Autodesk Inventor part; units mm, degrees
ref_plane "YZ Plane" through (0, 0, 0) normal (1, 0, 0) x (0, 1, 0)
ref_plane "XZ Plane" through (0, 0, 0) normal (0, 1, 0) x (-1, 0, 0)
ref_plane "XY Plane" through (0, 0, 0) normal (0, 0, 1) x (1, 0, 0)
sketch "Sketch1" plane through (0, 0, 0) normal (0, 0, 1) x (1, 0, 0)
  circle A0 centre (0, 0) radius 2.667
  circle A1 centre (0, 0) radius 4.167
  line L0 (-1.25, 3.9751) -> (1.25, 3.9751)
  line L1 (1.25, 3.9751) -> (1.25, 37.2251)
  line L2 (1.25, 37.2251) -> (-1.25, 37.2251)
  line L3 (-1.25, 37.2251) -> (-1.25, 3.9751)
  line L4 (0, 0) -> (0, 14.9208)
  circle A2 centre (0, 37.2251) radius 3
  circle A3 centre (0, 37.2251) radius 6
  line L5 (0, 43.2251) -> (6, 43.2251)
  line L6 (6, 43.2251) -> (6, 40.2251)
  line L7 (6, 40.2251) -> (0, 40.2251)
  point P0 (-1.25, 31.3567)
  point P1 (1.25, 3.9751)
  point P2 (1.25, 3.9751)
  point P3 (1.25, 34.4979)
  dimension "d1" = 8.334
  dimension "d5" = 6
  dimension "d6" = 12
  dimension "d0" = 5.334
  dimension "d2" = 1.25
  dimension "d3" = 1.25
  dimension "d4" = 33.25
  dimension "d7" = 6
extrude "Extrusion1" add sketch "Sketch1" along normal blind 2 contours L0 A1 | L0 A1 L4 | L4 A1 L0 | L3 A3 L1 A1 | A3 L7 A2 L3 | L3 A2 L1 A3 | L5 L6 L7 A3
fillet "Fillet1" radius 3.175 2 edges at (1.25, 34.4979, 1) (-1.25, 31.3567, 1)
equation "\"d2\" = d3"
properties part number "Hook"
CAD build for the part. Positions are in the model's coordinates, mm. A direction names the side the tool comes from. Round coordinates to 2 decimals unless told otherwise and drop trailing zeros. Write each loop counter-clockwise with the first axis right and the second up, starting at its lowest first coordinate (ties: lowest second). Pieces come first, ordered by that corner, then holes. Notation, with made-up numbers: M 44,32.5 L 62,32.5 A15 ccw 62,36.5 Z; hole C -10,38 d2. An arc over 180 degrees is marked long. Use a Markdown table: item, result. Add a question column.
1. Slice it at B-B on z = 0.45. Give the cut face in (x, y) (3 decimals), then the cut area to 3 significant figures.
2. 3-axis set-ups, long thin cutter, end or side, ignore diameter. For faces 5 (the face through (-1.25, 17, 1)), 6 (the face through (6, 42, 1)), 7 (the face through (3, 40.225, 1)): which of +Z, -Z, +X, -X, +Y, -Y reach the whole face in a straight line?
3. Slice it at A-A on y = 0. Give the cut face in (x, z).
4. Pull direction Y, two halves, no side cores. Call faces 1 (the face through (1.25, 17, 1)), 2 (the face through (1.231, 2.366, 0.986)), 3 (the face through (0, 21, 2)), 4 (the face through (3, 43.225, 1)): released by +Y, released by -Y, zero draft, split by the parting line, or undercut.
5. Flat gauge pin, fed straight in: P1, Ø0.6, axis at y = 19.5, z = 1, coming from the +X side. Where does the tip first touch, or does it go through?
6. Drill centre lines: probe 1 along X at (y, z) = (0, 0.45); probe 2 along Y at (x, z) = (1.5, 1.05); probe 3 along Y at (x, z) = (0, 0.6). Where is each one in solid material? Low to high.
7. Slice it at C-C on x = 2. Give the cut face in (y, z).
Reply:
| question | item | result |
|---|---|---|
| 1 | outline | M -2.894,31.969 A3.175 cw -1.25,29.188 L -1.25,3.975 A4.167 ccw long 1.25,3.975 L 1.25,31.358 A3.175 ccw -0.935,34.375 A3 cw 0,40.225 L 6,40.225 L 6,43.225 L 0,43.225 A6 ccw Z; hole C 0,0 d5.334 |
| 1 | area | 163 mm^2 |
| 2 | face 5 | +Z, -Z, -X |
| 2 | face 6 | +Z, -Z, +X, +Y, -Y |
| 2 | face 7 | +Z, -Z, +X |
| 3 | outline | M -4.17,0 L -2.67,0 L -2.67,2 L -4.17,2 Z; M 2.67,0 L 4.17,0 L 4.17,2 L 2.67,2 Z |
| 4 | face 1 | undercut |
| 4 | face 2 | undercut |
| 4 | face 3 | zero draft |
| 4 | face 4 | released by +Y |
| 5 | P1 | stops at x = 1.25 |
| 6 | probe 1 | x = -4.17 to -2.67, 2.67 to 4.17 |
| 6 | probe 2 | y = -3.89 to -2.21, 2.21 to 3.89, 40.23 to 43.23 |
| 6 | probe 3 | y = -4.17 to -2.67, 2.67 to 33.88, 40.23 to 43.23 |
| 7 | outline | M -3.66,0 L -1.76,0 L -1.76,2 L -3.66,2 Z; M 1.76,0 L 3.66,0 L 3.66,2 L 1.76,2 Z; M 40.23,0 L 43.23,0 L 43.23,2 L 40.23,2 Z |
